Autodesk Inventor part; units mm, degrees
ref_plane "YZ Plane" through (0, 0, 0) normal (1, 0, 0) x (0, 1, 0)
ref_plane "XZ Plane" through (0, 0, 0) normal (0, 1, 0) x (-1, 0, 0)
ref_plane "XY Plane" through (0, 0, 0) normal (0, 0, 1) x (1, 0, 0)
sketch "Sketch1" plane through (0, 0, 0) normal (0, 1, 0) x (-1, 0, 0)
  line L0 (50, 25) -> (-50, 25)
  line L1 (-50, 25) -> (-50, -25)
  line L2 (-50, -25) -> (50, -25)
  line L3 (50, -25) -> (50, 25)
  line L4 (50, 25) -> (-50, -25) construction
  line L5 (-50, 25) -> (50, -25) construction
  point P0 (0, 0)
  dimension "d0" = 100
  dimension "d1" = 50
extrude "Extrusion1" add sketch "Sketch1" along normal blind 6
fillet "Fillet1" radius 5 4 edges at (50, 3, 25) (50, 3, -25) (-50, 3, -25) (-50, 3, 25)
sketch "Sketch2" plane through (0, 6, 0) normal (0, 1, 0) x (1, 0, 0)
  line L0 (-39.5, -21.25) -> (-30.5, -21.25)
  line L1 (-30.5, -21.25) -> (-30.5, -4.75)
  line L2 (-30.5, -4.75) -> (-39.5, -4.75)
  line L3 (-39.5, -4.75) -> (-39.5, -21.25)
  line L4 (-39.5, -21.25) -> (-30.5, -4.75) construction
  line L5 (-30.5, -21.25) -> (-39.5, -4.75) construction
  line L6 (-25.5, -21.25) -> (-16.5, -21.25)
  line L7 (-16.5, -21.25) -> (-16.5, -4.75)
  line L8 (-16.5, -4.75) -> (-25.5, -4.75)
  line L9 (-25.5, -4.75) -> (-25.5, -21.25)
  line L10 (-25.5, -21.25) -> (-16.5, -4.75) construction
  line L11 (-16.5, -21.25) -> (-25.5, -4.75) construction
  line L12 (-11.5, -21.25) -> (-2.5, -21.25)
  line L13 (-2.5, -21.25) -> (-2.5, -4.75)
  line L14 (-2.5, -4.75) -> (-11.5, -4.75)
  line L15 (-11.5, -4.75) -> (-11.5, -21.25)
  line L16 (-11.5, -21.25) -> (-2.5, -4.75) construction
  line L17 (-2.5, -21.25) -> (-11.5, -4.75) construction
  line L18 (2.5, -21.25) -> (11.5, -21.25)
  line L19 (11.5, -21.25) -> (11.5, -4.75)
  line L20 (11.5, -4.75) -> (2.5, -4.75)
  line L21 (2.5, -4.75) -> (2.5, -21.25)
  line L22 (2.5, -21.25) -> (11.5, -4.75) construction
  line L23 (11.5, -21.25) -> (2.5, -4.75) construction
  line L24 (16.5, -21.25) -> (25.5, -21.25)
  line L25 (25.5, -21.25) -> (25.5, -4.75)
  line L26 (25.5, -4.75) -> (16.5, -4.75)
  line L27 (16.5, -4.75) -> (16.5, -21.25)
  line L28 (16.5, -21.25) -> (25.5, -4.75) construction
  line L29 (25.5, -21.25) -> (16.5, -4.75) construction
  line L30 (30.5, -21.25) -> (39.5, -21.25)
  line L31 (39.5, -21.25) -> (39.5, -4.75)
  line L32 (39.5, -4.75) -> (30.5, -4.75)
  line L33 (30.5, -4.75) -> (30.5, -21.25)
  line L34 (30.5, -21.25) -> (39.5, -4.75) construction
  line L35 (39.5, -21.25) -> (30.5, -4.75) construction
  line L36 (-45, -25) -> (45, -25)
  line L37 (-50, 20) -> (-50, -20)
  point P0 (0, 0)
  point P1 (-35, -13)
  point P2 (-21, -13)
  point P3 (-7, -13)
  point P4 (7, -13)
  point P5 (21, -13)
  point P6 (35, -13)
  dimension "d5" = 9
  dimension "d6" = 16.5
  dimension "d9" = 14
  dimension "d14" = 7
  dimension "d15" = 13
  dimension "d44" = 12
  dimension "d45" = 15
extrude "Extrusion2" cut sketch "Sketch2" against normal blind 10
sketch "Sketch3" plane through (0, 6, 0) normal (0, 1, 0) x (1, 0, 0)
  line L0 (-16.5, -21.25) -> (-25.5, -21.25)
  line L1 (-45, -25) -> (45, -25)
  line L2 (45, 25) -> (-45, 25)
  line L3 (-38, 0) -> (-32, 0)
  line L4 (-32, 0) -> (-32, 20)
  line L5 (-32, 20) -> (-38, 20)
  line L6 (-38, 20) -> (-38, 0)
  line L7 (-38, 0) -> (-32, 20) construction
  line L8 (-32, 0) -> (-38, 20) construction
  line L9 (-24, 0) -> (-18, 0)
  line L10 (-18, 0) -> (-18, 20)
  line L11 (-18, 20) -> (-24, 20)
  line L12 (-24, 20) -> (-24, 0)
  line L13 (-24, 0) -> (-18, 20) construction
  line L14 (-18, 0) -> (-24, 20) construction
  line L15 (-10, 0) -> (-4, 0)
  line L16 (-4, 0) -> (-4, 20)
  line L17 (-4, 20) -> (-10, 20)
  line L18 (-10, 20) -> (-10, 0)
  line L19 (-10, 0) -> (-4, 20) construction
  line L20 (-4, 0) -> (-10, 20) construction
  line L21 (4, 0) -> (10, 0)
  line L22 (10, 0) -> (10, 20)
  line L23 (10, 20) -> (4, 20)
  line L24 (4, 20) -> (4, 0)
  line L25 (4, 0) -> (10, 20) construction
  line L26 (10, 0) -> (4, 20) construction
  line L27 (18, 0) -> (24, 0)
  line L28 (24, 0) -> (24, 20)
  line L29 (24, 20) -> (18, 20)
  line L30 (18, 20) -> (18, 0)
  line L31 (18, 0) -> (24, 20) construction
  line L32 (24, 0) -> (18, 20) construction
  line L33 (32, 0) -> (38, 0)
  line L34 (38, 0) -> (38, 20)
  line L35 (38, 20) -> (32, 20)
  line L36 (32, 20) -> (32, 0)
  line L37 (32, 0) -> (38, 20) construction
  line L38 (38, 0) -> (32, 20) construction
  line L39 (-50, 20) -> (-50, -20)
  point P0 (0, 0)
  point P1 (-35, 10)
  point P2 (-21, 10)
  point P3 (-7, 10)
  point P4 (7, 10)
  point P5 (21, 10)
  point P6 (35, 10)
  dimension "d20" = 14
  dimension "d25" = 7
  dimension "d26" = 6
  dimension "d27" = 20
  dimension "d28" = 5
  dimension "d29" = 3.75
  dimension "d41" = 15
  dimension "d42" = 15
  dimension "d43" = 35
extrude "Extrusion3" cut sketch "Sketch3" against normal blind 10
sketch "Sketch4" plane through (0, 6, 0) normal (0, 1, 0) x (1, 0, 0)
  arc A0 (-50, -20) -> (-45, -25) centre (-45, -20) ccw
  arc A1 (45, -25) -> (50, -20) centre (45, -20) ccw
  arc A2 (50, 20) -> (45, 25) centre (45, 20) ccw
  arc A3 (-45, 25) -> (-50, 20) centre (-45, 20) ccw
  line L0 (45, 25) -> (-45, 25)
  line L1 (-50, 20) -> (-50, -20)
  point P0 (0, 0)
  dimension "d39" = 5
  dimension "d40" = 5
hole "Hole1" at (-45, 6, -20) at (45, 6, -20) at (45, 6, 20) at (-45, 6, 20) direction (0, -1, 0) diameter 4 end through all
properties part number "AcrylicUpperTop" material "Acrylic, Clear"
Model file for the job. Use its own axes, mm. A direction names the side the tool comes from. Coordinates: 2 decimals unless noted, no trailing zeros. Order: outer loops, then holes, each group sorted by start corner. A loop starts at its lowest first (then second) coordinate and runs counter-clockwise, first axis right, second up. Notation, with made-up numbers: (79.5, 69.25) - (120.5, 69.25) arc R27 cw to (120.5, 104.25) - close; hole circle Ø3 at (68, -39). An arc over 180 degrees is marked (long way). Return JSON: item names as keys, results as strings. Group by question number.
1) Mould opens along X. For faces 3 (the flat face through (25.5, 3, 13)), 4 (the flat face through (1, 6, 0)), 5 (the cylindrical face through (49, 3, -23)), 6 (the flat face through (-24, 3, -10)) say: released by +X, released by -X, zero draft, split by the parting line, or undercut.
2) Saw through at B-B, the plane x = 34. Write the cut outline in (y, z).
3) Saw through at C-C, the plane z = 14.5. Write the cut outline in (x, y), plus the area to 3 significant figures.
4) Probe line 1 (Z direction, x = -45, y = 3.45); line 2 (Z direction, x = 34.5, y = 5); line 3 (Z direction, x = -25, y = 4.9). List the from-to ranges inside material, lowest first. Write a range as from..to.
5) Tool access for faces 1 (the flat face through (10, 3, -10)), 2 (the flat face through (1, 0, 0)): list every direction of +Z, -Z, +X, -X, +Y, -Y with a clear straight run to the whole face (end or side of a thin tool).
6) Flat gauge pin, fed straight in: P1, Ø6, axis at x = -8, z = 13.5, coming from the -Y side. Where does the tip first touch, or does it go through?
7) Saw through at D-D, the plane y = 4.4. Count the separate pieces of the cut face and the enclosed holes in it, plus the area to 3 significant figures.
8) Saw through at A-A, the plane z = -16.5. Write the cut outline in (x, y).
Values found:
{
 "1": {"face 3": "undercut", "face 4": "zero draft", "face 5": "released by +X", "face 6": "undercut"},
 "2": {"outline": "(0, -25) - (6, -25) - (6, -20) - (0, -20) - close; (0, 0) - (6, 0) - (6, 4.75) - (0, 4.75) - close; (0, 21.25) - (6, 21.25) - (6, 25) - (0, 25) - close"},
 "3": {"outline": "(-50, 0) - (-39.5, 0) - (-39.5, 6) - (-50, 6) - close; (-30.5, 0) - (-25.5, 0) - (-25.5, 6) - (-30.5, 6) - close; (-16.5, 0) - (-11.5, 0) - (-11.5, 6) - (-16.5, 6) - close; (-2.5, 0) - (2.5, 0) - (2.5, 6) - (-2.5, 6) - close; (11.5, 0) - (16.5, 0) - (16.5, 6) - (11.5, 6) - close; (25.5, 0) - (30.5, 0) - (30.5, 6) - (25.5, 6) - close; (39.5, 0) - (50, 0) - (50, 6) - (39.5, 6) - close", "area": "276 mm²"},
 "4": {"line 1": "z = -25..-22, -18..18, 22..25", "line 2": "z = -25..-20, 0..4.75, 21.25..25", "line 3": "z = -25..4.75, 21.25..25"},
 "5": {"face 1": "+Y, -Y", "face 2": "+Z, -Z, +X, -X, -Y"},
 "6": {"P1": "passes through"},
 "7": {"separate pieces": "1", "enclosed holes": "16", "area": "3,320 mm²"},
 "8": {"outline": "(-50, 0) - (-38, 0) - (-38, 6) - (-50, 6) - close; (-32, 0) - (-24, 0) - (-24, 6) - (-32, 6) - close; (-18, 0) - (-10, 0) - (-10, 6) - (-18, 6) - close; (-4, 0) - (4, 0) - (4, 6) - (-4, 6) - close; (10, 0) - (18, 0) - (18, 6) - (10, 6) - close; (24, 0) - (32, 0) - (32, 6) - (24, 6) - close; (38, 0) - (50, 0) - (50, 6) - (38, 6) - close"}
}
